Check sheet for the modelled part. Datum: model origin and axes. Units: mm. Face numbers are marked on the shaded views. Round coordinates to 2 decimals unless told otherwise and drop trailing zeros. Loops run counter-clockwise (first coordinate to the right, second up) from the corner with the lowest first, then second, coordinate; pieces in that order, holes last. Notation, with made-up numbers: (56, 87.25) - (63, 87.25) arc R11 cw to (63, 92.25) - close; hole circle Ø6 at (-1.5, 59.5). An arc over 180 degrees is marked (long way). Put each result on its own line as item: value. Start each with the question number.
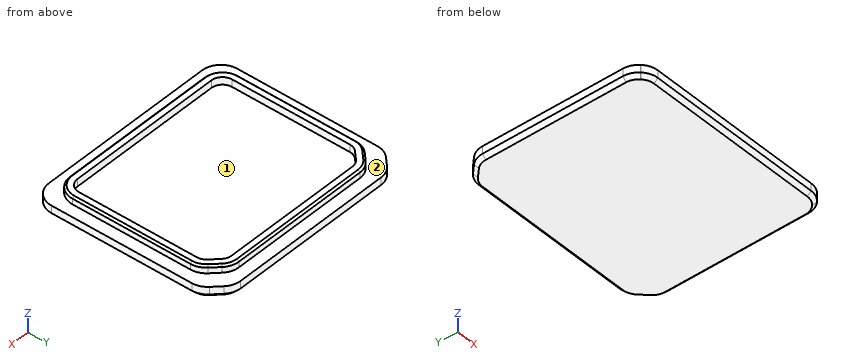
```python
from build123d import *

# Parameters (mm, degrees)
BOSS_EXTRUDE1_DEPTH = 3
BOSS_EXTRUDE2_DEPTH = 2
CHAMFER1_SIZE       = 1
FILLET1_R           = 3
FILLET2_R           = 5
CHAMFER2_SIZE       = 0.5


with BuildPart() as part:
    # Sketch2 → Boss-Extrude1 (new body)
    with BuildSketch(Plane(origin=(0, 0, -23.390463949), x_dir=(-1, 0, 0), z_dir=(0, 0, -1))):
        with BuildLine():
            Line((21.428932188, 26), (-22.307932188, 26))
            ThreePointArc((-22.307932188, 26), (-24.22134935, 25.619397663), (-25.843466094, 24.535533906))
            Line((-25.843466094, 24.535533906), (-27.914533906, 22.464466094))
            ThreePointArc((-27.914533906, 22.464466094), (-28.998397663, 20.84234935), (-29.379, 18.928932188))
            Line((-29.379, 18.928932188), (-29.379, -18.928932188))
            ThreePointArc((-29.379, -18.928932188), (-28.998397663, -20.84234935), (-27.914533906, -22.464466094))
            Line((-27.914533906, -22.464466094), (-27.843466094, -22.535533906))
            ThreePointArc((-27.843466094, -22.535533906), (-26.22134935, -23.619397663), (-24.307932188, -24))
            Line((-24.307932188, -24), (23.428932188, -24))
            ThreePointArc((23.428932188, -24), (25.34234935, -23.619397663), (26.964466094, -22.535533906))
            Line((26.964466094, -22.535533906), (27.035533906, -22.464466094))
            ThreePointArc((27.035533906, -22.464466094), (28.119397663, -20.84234935), (28.5, -18.928932188))
            Line((28.5, -18.928932188), (28.5, 18.928932188))
            ThreePointArc((28.5, 18.928932188), (28.119397663, 20.84234935), (27.035533906, 22.464466094))
            Line((27.035533906, 22.464466094), (24.964466094, 24.535533906))
            ThreePointArc((24.964466094, 24.535533906), (23.34234935, 25.619397663), (21.428932188, 26))
        make_face()
    extrude(amount=BOSS_EXTRUDE1_DEPTH)

    # Sketch3 → Boss-Extrude2 (add)
    with BuildSketch(Plane(origin=(0, 0, -23.390463949), x_dir=(-1, 0, 0), z_dir=(0, 0, -1))):
        Polygon((-26.279, -20.9), (25.4, -20.9), (25.4, 17.958578644), (20.458578644, 22.9), (-21.337578644, 22.9), (-26.279, 17.958578644), align=None)
        Polygon((-24.279, -18.9), (23.4, -18.9), (23.4, 17.130151519), (19.630151519, 20.9), (-20.509151519, 20.9), (-24.279, 17.130151519), align=None, mode=Mode.SUBTRACT)
    extrude(amount=-BOSS_EXTRUDE2_DEPTH)

    # Chamfer1
    chamfer1_edges = [part.edges().sort_by_distance(p)[0] for p in [
        (28.998397663, 20.84234935, -26.390463949),
        (29.379, 0, -26.390463949),
        (28.998397663, -20.84234935, -26.390463949),
        (27.879, -22.5, -26.390463949),
        (26.22134935, -23.619397663, -26.390463949),
        (0.4395, -24, -26.390463949),
        (-25.34234935, -23.619397663, -26.390463949),
        (-27, -22.5, -26.390463949),
        (-28.119397663, -20.84234935, -26.390463949),
        (-28.5, 0, -26.390463949),
        (24.22134935, 25.619397663, -26.390463949),
        (-28.119397663, 20.84234935, -26.390463949),
        (-26, 23.5, -26.390463949),
        (-23.34234935, 25.619397663, -26.390463949),
        (0.4395, 26, -26.390463949),
        (26.879, 23.5, -26.390463949),
    ]]
    chamfer(chamfer1_edges, length=CHAMFER1_SIZE)

    # Fillet1
    fillet1_edges = [part.edges().sort_by_distance(p)[0] for p in [
        (24.279, 17.130151519, -22.390463949),
        (20.509151519, 20.9, -22.390463949),
        (-19.630151519, 20.9, -22.390463949),
        (-23.4, 17.130151519, -22.390463949),
        (-23.4, -18.9, -22.390463949),
        (24.279, -18.9, -22.390463949),
    ]]
    fillet(fillet1_edges, radius=FILLET1_R)

    # Fillet2
    fillet2_edges = [part.edges().sort_by_distance(p)[0] for p in [
        (26.279, -20.9, -22.390463949),
        (26.279, 17.958578644, -22.390463949),
        (21.337578644, 22.9, -22.390463949),
        (-20.458578644, 22.9, -22.390463949),
        (-25.4, 17.958578644, -22.390463949),
        (-25.4, -20.9, -22.390463949),
    ]]
    fillet(fillet2_edges, radius=FILLET2_R)

    # Chamfer2
    chamfer2_edges = [part.edges().sort_by_distance(p)[0] for p in [
        (-25.4, -0.006244584, -21.390463949),
        (-22.929289322, 20.429289322, -21.390463949),
        (26.279, -0.006244584, -21.390463949),
        (23.808289322, 20.429289322, -21.390463949),
        (0.4395, 22.9, -21.390463949),
        (0.4395, -20.9, -21.390463949),
        (24.814533906, -19.435533906, -21.390463949),
        (-23.935533906, -19.435533906, -21.390463949),
        (25.898397663, 17.800927994, -21.390463949),
        (21.179927994, 22.519397663, -21.390463949),
        (-20.300927994, 22.519397663, -21.390463949),
        (-25.019397663, 17.800927994, -21.390463949),
    ]]
    chamfer(chamfer2_edges, length=CHAMFER2_SIZE)


solid = part.part
```
Q1. Cross-section at A-A on z = -22.6. Enter the section's corners in (x, y).
Q2. Depth check by flat-ended pin: pin 1 Ø25 at (x, y) = (10, 3.5) entering from +Z; pin 2 Ø2 at (y, z) = (0.5, -22.5) entering from +X; pin 3 Ø1.5 at (y, z) = (-2, -22) entering from -X; pin 4 Ø1.6 at (x, z) = (-4.5, -22.5) entering from +Y. Enter the tip coordinate at first touch or a pass-through.
Q3. Material ranges on line 1 (Y direction, x = 15, z = -23.2); line 2 (X direction, y = 1.5, z = -23.15); line 3 (Z direction, x = 24, y = 6), recorded low to high. Write a range as from..to.
Q4. Draft check along Y on the marked faces 1 and 2. Enter one of: +Y half, -Y half, draft (parallel to the pull), parting line (faces both ways), or undercut.
Q5. Cross-section at B-B on x = -14. Enter the section's corners in (y, z).
Q6. Cross-section at C-C on y = 5.5. Enter the section's corners in (x, z), and give its area (3 significant figures).
Answer list:
1. outline: (-25.4, -15.9) arc R5 ccw to (-20.4, -20.9) - (21.28, -20.9) arc R5 ccw to (26.28, -15.9) - (26.28, 15.89) arc R5 ccw to (24.81, 19.42) - (22.8, 21.44) arc R5 ccw to (19.27, 22.9) - (-18.39, 22.9) arc R5 ccw to (-21.92, 21.44) - (-23.94, 19.42) arc R5 ccw to (-25.4, 15.89) - close; hole (-23.4, -15.9) arc R3 ccw to (-20.4, -18.9) - (21.28, -18.9) arc R3 ccw to (24.28, -15.9) - (24.28, 15.89) arc R3 ccw to (23.4, 18.01) - (21.39, 20.02) arc R3 ccw to (19.27, 20.9) - (-18.39, 20.9) arc R3 ccw to (-20.51, 20.02) - (-22.52, 18.01) arc R3 ccw to (-23.4, 15.89) - close
2. pin 1: stops at z = -23.39
2. pin 2: stops at x = 29.38
2. pin 3: stops at x = -25.4
2. pin 4: stops at y = 22.9
3. line 1: y = -20.9..-18.9, 20.9..22.9
3. line 2: x = -25.4..-23.4, 24.28..26.28
3. line 3: z = -26.39..-23.39
4. face 1: undercut
4. face 2: draft
5. outline: (-24, -25.39) - (-23, -26.39) - (25, -26.39) - (26, -25.39) - (26, -23.39) - (22.9, -23.39) - (22.9, -21.89) - (22.4, -21.39) - (20.9, -21.39) - (20.9, -23.39) - (-18.9, -23.39) - (-18.9, -21.39) - (-20.4, -21.39) - (-20.9, -21.89) - (-20.9, -23.39) - (-24, -23.39) - close
6. outline: (-28.5, -25.39) - (-27.5, -26.39) - (28.38, -26.39) - (29.38, -25.39) - (29.38, -23.39) - (26.28, -23.39) - (26.28, -21.89) - (25.78, -21.39) - (24.28, -21.39) - (24.28, -23.39) - (-23.4, -23.39) - (-23.4, -21.39) - (-24.9, -21.39) - (-25.4, -21.89) - (-25.4, -23.39) - (-28.5, -23.39) - close
6. area: 180 mm2
